Could you check a few things on this model? Use its own coordinates, in mm. Round coordinates to 2 decimals unless told otherwise and drop trailing zeros. Order: outer loops, then holes, each group sorted by start corner. A loop starts at its lowest first (then second) coordinate and runs counter-clockwise, first axis right, second up. Notation, with made-up numbers: (3.25, 58) - (7.25, 58) arc R12 cw to (7.25, 78) - close; hole circle Ø8 at (-17.5, 33). An arc over 180 degrees is marked (long way). Return JSON: item names as keys, results as strings. Group by question number.
from build123d import *

# Parameters (mm, degrees)
F0_W     = 104
F0_H     = 80
F1_DEPTH = 1.5


with BuildPart() as f1:
    # F0 (on Front) → F1 (new body)
    with BuildSketch(Plane.XZ):
        Polygon((81.5, -86), (81.5, 86), (-81.5, 86), (-81.5, -86), (-3, -86), (3, -86), align=None)
        with Locations((0, 17.5)):
            Rectangle(F0_W, F0_H, mode=Mode.SUBTRACT)
    extrude(amount=F1_DEPTH)


solid = f1.part
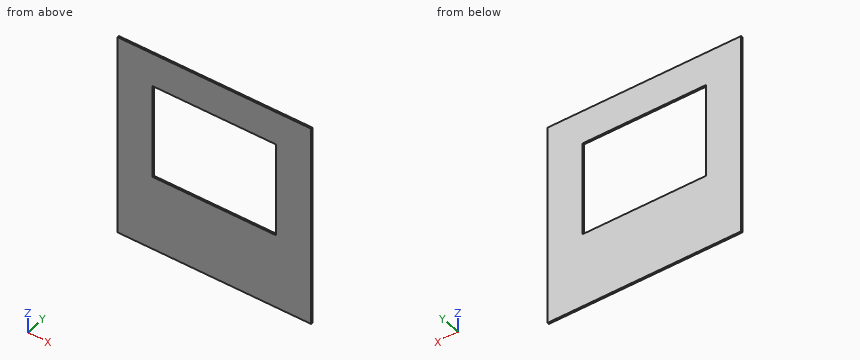
1) If I drill on line 1 along X through (y, z) = (-0.9, -16.5); line 2 along Z through (x, y) = (-39.5, -0.5), over which ranges is the centre line in solid material (lowest first)? Write a range as from..to.
2) I want a section at C-C, the plane y = -0.95. List the corners of the cut face in (x, z) for me, plus the area to 3 significant figures.
3) I want a section at B-B, the plane x = -49.5. List the corners of the cut face in (y, z) for me.
4) I want a section at A-A, the plane z = -5. List the corners of the cut face in (x, y) for me.
Outcome:
{
 "1": {"line 1": "-81.5..-52, 52..81.5", "line 2": "-86..-22.5, 57.5..86"},
 "2": {"outline": "(-81.5, -86) - (81.5, -86) - (81.5, 86) - (-81.5, 86) - close; hole (-52, -22.5) - (52, -22.5) - (52, 57.5) - (-52, 57.5) - close", "area": "19,700 mm^2"},
 "3": {"outline": "(-1.5, -86) - (0, -86) - (0, -22.5) - (-1.5, -22.5) - close; (-1.5, 57.5) - (0, 57.5) - (0, 86) - (-1.5, 86) - close"},
 "4": {"outline": "(-81.5, -1.5) - (-52, -1.5) - (-52, 0) - (-81.5, 0) - close; (52, -1.5) - (81.5, -1.5) - (81.5, 0) - (52, 0) - close"}
}
